For this review, take the finished solid that the model builds, in its own axes (mm). A direction names the side the tool comes from. Give positions to 0.01 mm unless a question says otherwise; leave off trailing zeros. Order: outer loops, then holes, each group sorted by start corner. A loop starts at its lowest first (then second) coordinate and runs counter-clockwise, first axis right, second up. Notation, with made-up numbers: (-20.5, 17) -> (4.5, 17) arc R15 ccw to (4.5, 41) -> close; hole circle Ø5 at (33, -39). An arc over 180 degrees is marked (long way). One line per item, written item: value. Start each with the question number.
Autodesk Inventor part; units mm, degrees
ref_plane "YZ Plane" through (0, 0, 0) normal (1, 0, 0) x (0, 1, 0)
ref_plane "XZ Plane" through (0, 0, 0) normal (0, 1, 0) x (-1, 0, 0)
ref_plane "XY Plane" through (0, 0, 0) normal (0, 0, 1) x (1, 0, 0)
sketch "Sketch1" plane through (0, 0, 0) normal (0, 1, 0) x (-1, 0, 0)
  line L0 (10, 0) -> (0, 0)
  line L1 (0, 0) -> (0, -48)
  line L2 (0, -48) -> (10, -48)
  line L3 (10, -48) -> (10, 0)
  circle A0 centre (5, -7) radius 2.5
  circle A1 centre (5, -24) radius 2.5
  circle A2 centre (5, -41) radius 2.5
  circle A3 centre (5, -7) radius 3
  circle A4 centre (5, -24) radius 3
  circle A5 centre (5, -41) radius 3
  line L4 (5, -16) -> (5, -46.75) construction
  line L5 (8.25, -33.75) -> (1.75, -33.75)
  line L6 (1.75, -31.25) -> (8.25, -31.25)
  line L7 (6.1849, -32.5) -> (1.6849, -32.5) construction
  line L8 (8.25, -31.25) -> (8.25, -33.75)
  line L9 (1.75, -31.25) -> (1.75, -33.75)
  dimension "d0" = 48
  dimension "d1" = 10
  dimension "d4" = 5
  dimension "d24" = 6
  dimension "d48" = 7
  dimension "d49" = 24
  dimension "d50" = 41
  dimension "d51" = 2.5
  dimension "d52" = 15.5
  dimension "d53" = 6.5
extrude "Extrusion1" add sketch "Sketch1" against normal blind 1.4 contours L3 L2 L1 L0 | A0 | A1 | A2 | A3 | A4 | A5 | L5 L9 L6 L8
extrude "Extrusion5" add sketch "Sketch1" along normal blind 8 contours A0
extrude "Extrusion6" add sketch "Sketch1" along normal blind 1 contours A3
fillet "Fillet4" radius 2.5 1 edges at (-2.5, 8, -7)
extrude "Extrusion7" add sketch "Sketch1" along normal blind 1 contours A4
extrude "Extrusion8" add sketch "Sketch1" along normal blind 8 contours A1
fillet "Fillet5" radius 2.5 1 edges at (-2.5, 8, -24)
extrude "Extrusion9" add sketch "Sketch1" along normal blind 8 contours A2
extrude "Extrusion10" add sketch "Sketch1" along normal blind 1 contours A5
fillet "Fillet6" radius 2.5 1 edges at (-2.5, 8, -41)
sketch "Sketch2" plane through (-5, 8, -24) normal (0, 1, 0) x (1, 0, 0)
  point P0 (0, 0)
sketch "Sketch3" plane through (0, -1.4, 0) normal (0, -1, 0) x (1, 0, 0)
  line L0 (-5, -16) -> (-5, -46.75) construction
  line L1 (-6.1849, -32.5) -> (-1.6849, -32.5) construction
  line L2 (-12.75, -29.75) -> (2.75, -29.75)
  line L3 (2.75, -29.75) -> (2.75, -35.25)
  line L4 (2.75, -35.25) -> (-12.75, -35.25)
  line L5 (-12.75, -35.25) -> (-12.75, -29.75)
  point P0 (0, 0)
  dimension "d56" = 15.5
  dimension "d57" = 5.5
extrude "Extrusion12" add sketch "Sketch3" along normal blind 5.5
extrude "Extrusion13" add sketch "Sketch1" along normal blind 1.5 contours L5 L9 L6 L8
properties part number "Led_Board_V1"
Q1. Take a section at A-A (z = -7). State the section outline as (x, y) points, and give its area (3 significant figures).
Q2. Take a section at C-C (x = -1.25). State the section outline as (y, z) points.
Q3. For pin 1 Ø5 at (x, y) = (-5.5, 6) entering from -Z; pin 2 Ø1 at (x, z) = (1, -33) entering from +Y; pin 3 Ø3 at (x, z) = (1, -33) entering from +Y, all flat-tipped, find the tip position at first contact; note any pin that passes through.
Q4. For faces 4 (the flat face through (-5, 1, -31.25)), 5 (the cylindrical face through (-6.34, 3.22, -26.11)), 6 (the flat face through (-8.25, 1, -32)), list the 3-axis set-ups (+Z, -Z, +X, -X, +Y, -Y) from which the entire face can be reached by the end or side of a thin tool; tool diameter is ignored.
Q5. Take a section at B-B (y = 5). State the section outline as (x, z) points, and give its area (3 significant figures).
Q6. Mouldability with a two-part tool opening along Z and no side actions: class faces 1 (the flat face through (-5, -1.4, -42)), 2 (the flat face through (-5, -4, -29.75)), 3 (the flat face through (-3, 1, -39)) as pulls with the +Z half, pulls with the -Z half, needs draft (parallel to the pull), parting line crosses it, or undercut.
Q7. For line 1 along Y through (x, z) = (-2.5, -3); line 2 along Z through (x, y) = (-10, -1.5); line 3 along Z through (x, y) = (-3.5, 7), list the stretches that pass through material, from the lowest coordinate up.
Q8. Take a section at D-D (z = -22). State the section outline as (x, y) points, and give its area (3 significant figures).
Answers below:
1. outline: (-10, -1.4) -> (0, -1.4) -> (0, 0) -> (-2, 0) -> (-2, 1) -> (-2.5, 1) -> (-2.5, 5.5) arc R2.5 ccw to (-7.5, 5.5) -> (-7.5, 1) -> (-8, 1) -> (-8, 0) -> (-10, 0) -> close
1. area: 52.3 mm²
2. outline: (-6.9, -35.25) -> (-1.4, -35.25) -> (-1.4, -48) -> (0, -48) -> (0, 0) -> (-1.4, 0) -> (-1.4, -29.75) -> (-6.9, -29.75) -> close
3. pin 1: stops at z = -43.5
3. pin 2: stops at y = -1.4
3. pin 3: stops at y = 0
4. face 4: +X, -X, +Y
4. face 5: +Y
4. face 6: +Z, -Z, -X, +Y
5. outline: circle Ø5 at (-5, -41); circle Ø5 at (-5, -24); circle Ø5 at (-5, -7)
5. area: 58.9 mm²
6. face 1: needs draft
6. face 2: pulls with the +Z half
6. face 3: undercut
7. line 1: y = -1.4 to 0
7. line 2: z = -35.25 to -29.75
7. line 3: z = -42.32 to -39.68, -25.32 to -22.68, -8.32 to -5.68
8. outline: (-10, -1.4) -> (0, -1.4) -> (0, 0) -> (-2.76, 0) -> (-2.76, 1) -> (-3.5, 1) -> (-3.5, 5.5) arc R1.5 ccw to (-6.5, 5.5) -> (-6.5, 1) -> (-7.24, 1) -> (-7.24, 0) -> (-10, 0) -> close
8. area: 35.5 mm²
